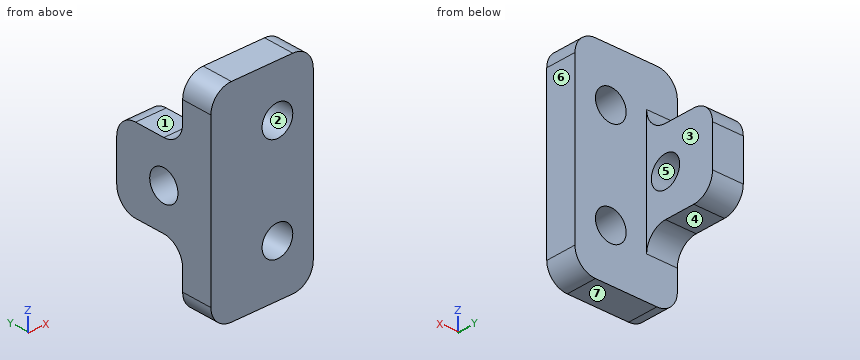
from build123d import *

# Parameters (mm, degrees)
SKETCH1_R           = 1.5
BOSS_EXTRUDE1_DEPTH = 3
SKETCH2_W           = 20
SKETCH2_H           = 3
BOSS_EXTRUDE2_DEPTH = 7
SKETCH3_R           = 1.5
CUT_EXTRUDE1_DEPTH  = 12.5
FILLET1_R           = 2


with BuildPart() as part:
    # Sketch1 → Boss-Extrude1 (new body)
    with BuildSketch(Plane(origin=(0, 0, 0), x_dir=(0, 0, -1), z_dir=(1, 0, 0))):
        Polygon((14, 10), (14, 3), (20, 3), (20, 0), (0, 0), (0, 3), (6, 3), (6, 10), align=None)
        with Locations((10, 5)):
            Circle(SKETCH1_R, mode=Mode.SUBTRACT)
    extrude(amount=BOSS_EXTRUDE1_DEPTH)

    # Sketch2 → Boss-Extrude2 (add)
    with BuildSketch(Plane(origin=(3, 0, 0), x_dir=(0, 0, -1), z_dir=(1, 0, 0))):
        with Locations((10, 1.5)):
            Rectangle(SKETCH2_W, SKETCH2_H)
    extrude(amount=BOSS_EXTRUDE2_DEPTH)

    # Sketch3 → Cut-Extrude1 (cut, symmetric)
    with BuildSketch(Plane(origin=(0, 3, 0), x_dir=(1, 0, 0), z_dir=(0, 1, 0))):
        with Locations(Location((6.5, 15, 0), (0, 0, 270))):
            Circle(SKETCH3_R)
        with Locations(Location((6.5, 5, 0), (0, 0, 270))):
            Circle(SKETCH3_R)
    extrude(amount=CUT_EXTRUDE1_DEPTH, both=True, mode=Mode.SUBTRACT)

    # Fillet1
    fillet1_edges = [part.edges().sort_by_distance(p)[0] for p in [
        (0, 1.5, -20),
        (0, 1.5, 0),
        (1.5, 3, -6),
        (1.5, 10, -6),
        (1.5, 10, -14),
        (1.5, 3, -14),
        (10, 1.5, 0),
        (10, 1.5, -20),
    ]]
    fillet(fillet1_edges, radius=FILLET1_R)


solid = part.part
Geometry check sheet. Reference: the model listing, model coordinates, mm. Face numbers are marked on the shaded views. A direction names the side the tool comes from. Round coordinates to 2 decimals unless told otherwise and drop trailing zeros. Write each loop counter-clockwise with the first axis right and the second up, starting at its lowest first coordinate (ties: lowest second). Pieces come first, ordered by that corner, then holes. Notation, with made-up numbers: (-24, 7) -> (7, 7) arc R30 cw to (7, 30) -> close; hole circle Ø5 at (36, -22.5). An arc over 180 degrees is marked (long way). One line per item, written item: value. Start each with the question number.
(1) Draft check along Z on the marked faces 5, 6 and 7. Enter one of: +Z half, -Z half, draft (parallel to the pull), parting line (faces both ways), or undercut.
(2) Go/stop test with flat-tipped pins: pin 1 Ø1 at (x, y) = (3, 7) entering from +Z; pin 2 Ø3 at (x, z) = (7.5, -13) entering from +Y; pin 3 Ø1.5 at (x, y) = (1, 6.5) entering from -Z. Record where each tip stops, or that it passes through.
(3) Cross-section at B-B, the plane z = -10. Record the cut outline in (x, y).
(4) Cross-section at C-C, the plane y = 2.75. Record the cut outline in (x, z).
(5) Scan lines: line 1 (X direction, y = 1.35, z = -5); line 2 (Z direction, x = 5.25, y = 2.75); line 3 (Y direction, x = 3.5, z = -4). Record each from-to range of solid material in increasing order. Write a range as [from, to].
(6) Cross-section at A-A, the plane x = 6.5. Record the cut outline in (y, z), and give its area (3 significant figures).
(7) Cross-section at D-D, the plane y = 6. Record the cut outline in (x, z), and give its area (3 significant figures).
(8) Access from +Z, -Z, +X, -X, +Y, -Y to the whole of each face (thin tool, end or side, straight path). Record for the marked faces 1, 2, 3 and 4.
Answer:
1. face 5: undercut
1. face 6: draft
1. face 7: -Z half
2. pin 1: z = -6
2. pin 2: y = 3
2. pin 3: z = -14
3. outline: (0, 0) -> (10, 0) -> (10, 3) -> (3, 3) -> (3, 3.5) -> (0, 3.5) -> close; (0, 6.5) -> (3, 6.5) -> (3, 10) -> (0, 10) -> close
4. outline: (0, -18) arc R2 ccw to (2, -20) -> (8, -20) arc R2 ccw to (10, -18) -> (10, -2) arc R2 ccw to (8, 0) -> (2, 0) arc R2 ccw to (0, -2) -> close; hole circle Ø3 at (6.5, -15); hole circle Ø3 at (6.5, -5)
5. line 1: [0, 5], [8, 10]
5. line 2: [-20, -15.83], [-14.17, -5.83], [-4.17, 0]
5. line 3: [0, 3]
6. outline: (0, -20) -> (3, -20) -> (3, -16.5) -> (0, -16.5) -> close; (0, -13.5) -> (3, -13.5) -> (3, -6.5) -> (0, -6.5) -> close; (0, -3.5) -> (3, -3.5) -> (3, 0) -> (0, 0) -> close
6. area: 42.0 mm²
7. outline: (0, -14) -> (3, -14) -> (3, -11.12) -> (0, -11.12) -> close; (0, -8.88) -> (3, -8.88) -> (3, -6) -> (0, -6) -> close
7. area: 17.3 mm²
8. face 1: +Z, +X, -X, +Y
8. face 2: +Y, -Y
8. face 3: +Z, -Z, +X, +Y
8. face 4: -Z, +X, -X, +Y
